```python
from build123d import *

# Parameters (mm, degrees)
F0_W      = 2000
F0_H      = 500
F1_DEPTH  = 1500
F2_R      = 141.1964442428
F3_DEPTH  = 100
F4_R      = 34.4012155817
F1_FACE_W = 2000
F1_FACE_H = 500
F1_FACE_R = 141.1964442428
F5_DEPTH  = 300
F6_R      = 22.2612942047
F7_DEPTH  = 25
F11_DEPTH = 25
F12_DEPTH = 500
F13_R     = 126.398375951
F14_DEPTH = 600


# Not quite as in the source:
# - a feature of the source that left no trace in its solid (it failed there, or was rolled back) is left out


with BuildPart() as f1:
    # F0 (on Top) → F1 (new body)
    with BuildSketch(Plane.XY):
        with Locations((-90.5123054981, -534.5377490795)):
            Rectangle(F0_W, F0_H)
    extrude(amount=-F1_DEPTH)

    # F2 (on Top) → F3 (cut)
    with BuildSketch(Plane.XY):
        with Locations((-797.8549599648, -524.8737335205)):
            Circle(F2_R)
    extrude(amount=-F3_DEPTH, mode=Mode.SUBTRACT)

    # F4 (on face) + F1_face (on face) → F5 (cut)
    with BuildSketch(Plane.XY.offset(-100)):
        with Locations((-826.4881968498, -472.618997097)):
            Circle(F4_R)
    with BuildSketch(Plane(origin=(-43.2497509657, -535.1834701589, 0), x_dir=(1, 0, 0), z_dir=(0, 0, 1))):
        with Locations((-47.2625545324, 0.6457210794)):
            Rectangle(F1_FACE_W, F1_FACE_H)
        with Locations((-754.605208999, 10.3097366384)):
            Circle(F1_FACE_R, mode=Mode.SUBTRACT)
    extrude(amount=F5_DEPTH, mode=Mode.SUBTRACT)

    # F6 (on Top) → F7 (cut)
    with BuildSketch(Plane.XY):
        with Locations((-837.3667597771, -527.3413062096)):
            Circle(F6_R)
    extrude(amount=-F7_DEPTH, mode=Mode.SUBTRACT)

    # F10 (on Top) → F11 (join)
    with BuildSketch(Plane.XY):
        with BuildLine():
            ThreePointArc((-336.3280592399, -643.7038848361), (-311.8886426753, -604.522487328), (-303.3533888527, -559.1394901276))
            ThreePointArc((-303.3533888527, -559.1394901276), (-314.3656518823, -507.8553931627), (-345.4608968402, -465.6130651073))
            ThreePointArc((-345.4608968402, -465.6130651073), (-373.9207280875, -556.3521241934), (-336.3280592399, -643.7038848361))
        make_face()
        with BuildLine():
            ThreePointArc((-345.4608968402, -465.6130651073), (-314.3656518823, -507.8553931627), (-303.3533888527, -559.1394901276))
            ThreePointArc((-303.3533888527, -559.1394901276), (-311.8886426753, -604.522487328), (-336.3280592399, -643.7038848361))
            ThreePointArc((-336.3280592399, -643.7038848361), (-266.2138077643, -683.0061743425), (-186.1307836251, -676.1223189436))
            ThreePointArc((-186.1307836251, -676.1223189436), (-169.5365195374, -576.3659050684), (-113.0004686355, -492.5185040457))
            ThreePointArc((-113.0004686355, -492.5185040457), (-221.6444367274, -413.5213420531), (-345.4608968402, -465.6130651073))
        make_face()
        with BuildLine():
            ThreePointArc((-336.3280592399, -643.7038848361), (-373.9207280875, -556.3521241934), (-345.4608968402, -465.6130651073))
            ThreePointArc((-345.4608968402, -465.6130651073), (-553.0316980704, -565.5372770485), (-336.3280592399, -643.7038848361))
        make_face()
        with BuildLine():
            ThreePointArc((289.3120863194, -664.3842458725), (144.8913865697, -445.641688806), (-113.0004686355, -492.5185040457))
            ThreePointArc((-113.0004686355, -492.5185040457), (-103.7589334647, -520.2685961551), (-100.6307099798, -549.3493080139))
            ThreePointArc((-100.6307099798, -549.3493080139), (-124.0033138355, -625.8046199509), (-186.1307836251, -676.1223189436))
            ThreePointArc((-186.1307836251, -676.1223189436), (57.3165773299, -902.1781192905), (289.3120863194, -664.3842458725))
        make_face()
        with BuildLine():
            ThreePointArc((-100.6307099798, -549.3493080139), (-103.7589334647, -520.2685961551), (-113.0004686355, -492.5185040457))
            ThreePointArc((-113.0004686355, -492.5185040457), (-169.5365195374, -576.3659050684), (-186.1307836251, -676.1223189436))
            ThreePointArc((-186.1307836251, -676.1223189436), (-124.0033138355, -625.8046199509), (-100.6307099798, -549.3493080139))
        make_face()
    extrude(amount=F11_DEPTH)

    # F12 (cut): a face of the model
    f12_faces = [f1.faces().sort_by_distance(p)[0] for p in [
        (-80.6836957397, -625.9699801923, 25),
    ]]
    extrude(f12_faces, amount=-F12_DEPTH, mode=Mode.SUBTRACT)

    # F13 (on Top) → F14 (cut)
    with BuildSketch(Plane.XY):
        with Locations((34.1630466282, -737.5611066818)):
            Circle(F13_R)
    extrude(amount=-F14_DEPTH, mode=Mode.SUBTRACT)


solid = f1.part
```
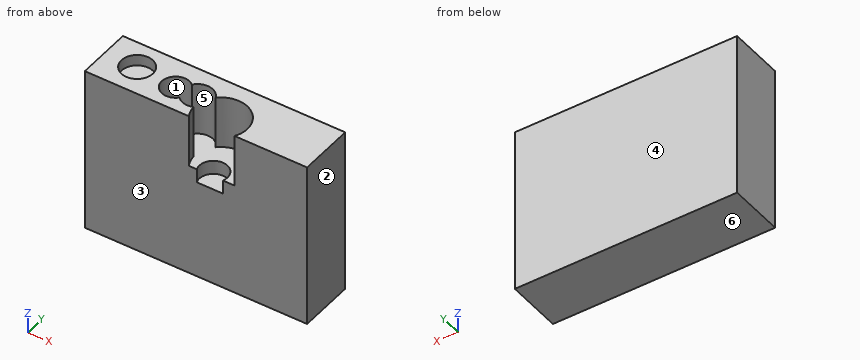
Source: CAD feature listing. Evaluate the final solid. Frame: model axes, mm. Face numbers are marked on the shaded views. A direction names the side the tool comes from. Coordinates: 2 decimals unless noted, no trailing zeros. Loops run counter-clockwise (first coordinate to the right, second up) from the corner with the lowest first, then second, coordinate; pieces in that order, holes last. Notation, with made-up numbers: (37.25, 59.25) -> (44.25, 59.25) arc R17 cw to (44.25, 64.25) -> close; hole circle Ø5 at (19.5, -27). An arc over 180 degrees is marked (long way). One line per item, written item: value. Start each with the question number.
Q1. Section query C-C, the plane y = -581. Return the cut outline in (x, z).
Q2. Mould query, pull axis Y, two halves, no side actions, for the marked faces 1, 2, 3 and 4. Classes: pulls with the +Y half, pulls with the -Y half, needs draft (parallel to the pull), parting line crosses it, or undercut.
Q3. Section query D-D, the plane y = -737.5. Return the cut outline in (x, z), and give its area (3 significant figures).
Q4. Section query A-A, the plane x = -7. Return the cut outline in (y, z), and give its area (3 significant figures).
Q5. Section query B-B, the plane z = -183. Return the cut outline in (x, y).
Q6. Set-up query: the marked faces 5 and 6. Return all of +Z, -Z, +X, -X, +Y, -Y with unobstructed straight access to the full face (end or side cutting, diameter ignored); none if empty.
Q7. Contact query for flat-ended pins moving along their axis: P1, Ø4, axis at x = 135.5, y = -490, coming from the +Z side; P2, Ø12, axis at x = 589.5, y = -481, coming from the +Z side; P3, Ø8, axis at x = -768, y = -559.5, coming from the +Z side. Output: stop coordinate, or through.
Q8. Line query: line 1 along X through (y, z) = (-609, -67.5); line 2 along Z through (x, y) = (177, -656.5); line 3 along Y through (x, z) = (-195, -128). Output: solid intervals per line, ascending.
Results:
1. outline: (-1090.51, -1500) -> (909.49, -1500) -> (909.49, 0) -> (274.22, 0) -> (274.22, -475) -> (-551.27, -475) -> (-551.27, 0) -> (-668.29, 0) -> (-668.29, -100) -> (-927.42, -100) -> (-927.42, 0) -> (-1090.51, 0) -> close
2. face 1: undercut
2. face 2: needs draft
2. face 3: pulls with the -Y half
2. face 4: pulls with the +Y half
3. outline: (-1090.51, -1500) -> (909.49, -1500) -> (909.49, 0) -> (277.8, 0) -> (277.8, -475) -> (160.56, -475) -> (160.56, -600) -> (-92.24, -600) -> (-92.24, -475) -> (-174.9, -475) -> (-174.9, 0) -> (-1090.51, 0) -> close
3. area: 2,750,000 mm^2
4. outline: (-784.54, -1500) -> (-284.54, -1500) -> (-284.54, 0) -> (-433.81, 0) -> (-433.81, -475) -> (-618.05, -475) -> (-618.05, -600) -> (-784.54, -600) -> close
4. area: 563,000 mm^2
5. outline: (-1090.51, -784.54) -> (-153.84, -784.54) arc R237.87 cw to (-186.13, -676.12) arc R136.73 cw to (-336.33, -643.7) arc R124.92 cw (long way) to (-345.46, -465.61) arc R136.73 cw to (-113, -492.52) arc R237.87 cw to (256.73, -784.54) -> (909.49, -784.54) -> (909.49, -284.54) -> (-1090.51, -284.54) -> close
6. face 5: +Z
6. face 6: -Z, +X, -X, +Y, -Y
7. P1: z = -475
7. P2: z = 0
7. P3: z = -100
8. line 1: -1090.51 to -911.25, -684.46 to -542.81, 282.77 to 909.49
8. line 2: -1500 to -475
8. line 3: -784.54 to -679.36, -419.34 to -284.54
